from build123d import *

# Parameters (mm, degrees)
SKETCH1_W           = 3
SKETCH1_H           = 3
SKETCH1_H_2         = 54.4
SKETCH1_W_2         = 30.6
SKETCH1_W_3         = 5.5
SKETCH1_W_4         = 13.6
SKETCH1_W_5         = 18
BOSS_EXTRUDE3_DEPTH = 3
SKETCH1_9_W         = 5.5
SKETCH1_9_H         = 3
SKETCH1_9_W_2       = 13.6
SKETCH1_9_W_3       = 18
SKETCH1_9_W_4       = 3
SKETCH1_9_H_2       = 54.4
SKETCH1_9_W_5       = 30.6
BOSS_EXTRUDE4_DEPTH = 15
CUT_EXTRUDE1_DEPTH  = 3
CUT_EXTRUDE2_DEPTH  = 3
SKETCH4_W           = 13.6
SKETCH4_H           = 11
CUT_EXTRUDE3_DEPTH  = 3
CUT_EXTRUDE4_DEPTH  = 3


with BuildPart() as part:
    # Sketch1 → Boss-Extrude3 (new body)
    with BuildSketch(Plane.XY):
        with Locations((1.5, 58.9)):
            Rectangle(SKETCH1_W, SKETCH1_H)
        with Locations((1.5, 30.2)):
            Rectangle(SKETCH1_W, SKETCH1_H_2)
        Polygon((0, 3), (0, 0), (76.2, 0), (76.2, 3), (3, 3), align=None)
        Polygon((3, 3), (76.2, 3), (76.2, 46.2), (58.2, 46.2), (58.2, 29), (52.7, 29), (52.7, 61.4), (39.1, 61.4), (39.1, 29), (33.6, 29), (33.6, 57.4), (3, 57.4), align=None)
        with Locations((18.3, 58.9)):
            Rectangle(SKETCH1_W_2, SKETCH1_H)
        Polygon((33.6, 60.4), (33.6, 57.4), (33.6, 29), (39.1, 29), (39.1, 61.4), (33.6, 61.4), align=None)
        with Locations((36.35, 62.9)):
            Rectangle(SKETCH1_W_3, SKETCH1_H)
        with Locations((45.9, 62.9)):
            Rectangle(SKETCH1_W_4, SKETCH1_H)
        with Locations((55.45, 62.9)):
            Rectangle(SKETCH1_W_3, SKETCH1_H)
        Polygon((58.2, 29), (58.2, 46.2), (58.2, 49.2), (58.2, 61.4), (52.7, 61.4), (52.7, 29), align=None)
        with Locations((67.2, 47.7)):
            Rectangle(SKETCH1_W_5, SKETCH1_H)
        with Locations((77.7, 47.7)):
            Rectangle(SKETCH1_W, SKETCH1_H)
        Polygon((76.2, 3), (76.2, 0), (79.2, 0), (79.2, 46.2), (76.2, 46.2), align=None)
    extrude(amount=BOSS_EXTRUDE3_DEPTH)

    # Sketch1_9 → Boss-Extrude4 (add)
    with BuildSketch(Plane.XY):
        Polygon((33.6, 60.4), (33.6, 57.4), (33.6, 29), (39.1, 29), (39.1, 61.4), (33.6, 61.4), align=None)
        with Locations((36.35, 62.9)):
            Rectangle(SKETCH1_9_W, SKETCH1_9_H)
        with Locations((45.9, 62.9)):
            Rectangle(SKETCH1_9_W_2, SKETCH1_9_H)
        with Locations((55.45, 62.9)):
            Rectangle(SKETCH1_9_W, SKETCH1_9_H)
        Polygon((58.2, 29), (58.2, 46.2), (58.2, 49.2), (58.2, 61.4), (52.7, 61.4), (52.7, 29), align=None)
        with Locations((67.2, 47.7)):
            Rectangle(SKETCH1_9_W_3, SKETCH1_9_H)
        with Locations((77.7, 47.7)):
            Rectangle(SKETCH1_9_W_4, SKETCH1_9_H)
        Polygon((76.2, 3), (76.2, 0), (79.2, 0), (79.2, 46.2), (76.2, 46.2), align=None)
        Polygon((0, 3), (0, 0), (76.2, 0), (76.2, 3), (3, 3), align=None)
        with Locations((1.5, 30.2)):
            Rectangle(SKETCH1_9_W_4, SKETCH1_9_H_2)
        with Locations((18.3, 58.9)):
            Rectangle(SKETCH1_9_W_5, SKETCH1_9_H)
        with Locations((1.5, 58.9)):
            Rectangle(SKETCH1_9_W_4, SKETCH1_9_H)
    extrude(amount=-BOSS_EXTRUDE4_DEPTH)

    # Sketch2 → Cut-Extrude1 (cut)
    with BuildSketch(Plane(origin=(0, 0, 0), x_dir=(-1, 0, 0), z_dir=(0, -1, 0))):
        Polygon((0, 0), (0, 15), (-33.6, 15), (-18.6, 0), align=None)
    extrude(amount=-CUT_EXTRUDE1_DEPTH, mode=Mode.SUBTRACT)

    # Sketch3 → Cut-Extrude2 (cut)
    with BuildSketch(Plane.ZY):
        Polygon((0, 3), (-15, 18), (-15, 3), align=None)
    extrude(amount=-CUT_EXTRUDE2_DEPTH, mode=Mode.SUBTRACT)

    # Sketch4 → Cut-Extrude3 (cut)
    with BuildSketch(Plane(origin=(0, 64.4, 0), x_dir=(1, 0, 0), z_dir=(0, 1, 0))):
        with Locations((45.9, 9.5)):
            Rectangle(SKETCH4_W, SKETCH4_H)
    extrude(amount=-CUT_EXTRUDE3_DEPTH, mode=Mode.SUBTRACT)

    # Sketch5 → Cut-Extrude4 (cut)
    with BuildSketch(Plane(origin=(0, 0, 0), x_dir=(-1, 0, 0), z_dir=(0, -1, 0))):
        Polygon((-33.6, 15), (-51.6, 15), (-36.6, 0), (-18.6, 0), align=None)
    extrude(amount=-CUT_EXTRUDE4_DEPTH, mode=Mode.SUBTRACT)


solid = part.part
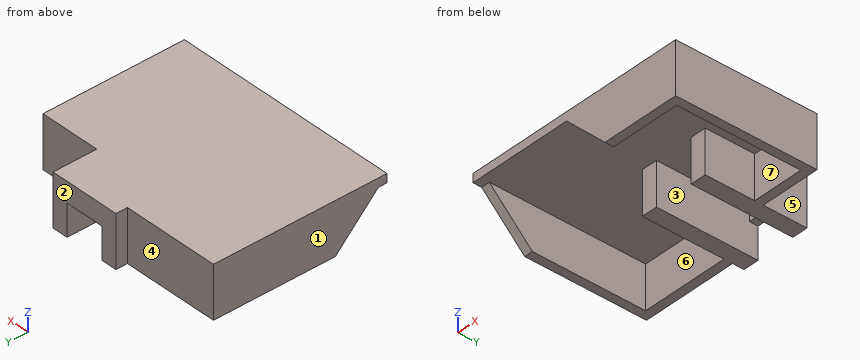
Verification items for the finished model (mm, model axes). Face numbers are marked on the shaded views. A direction names the side the tool comes from. Coordinates: 2 decimals unless noted, no trailing zeros. Order: outer loops, then holes, each group sorted by start corner. A loop starts at its lowest first (then second) coordinate and runs counter-clockwise, first axis right, second up. Notation, with made-up numbers: M 58,-30.5 L 65,-30.5 A15 cw 65,-2.5 Z; hole C 51.25,36.5 d2. An arc over 180 degrees is marked long. Return JSON: item names as keys, results as strings.
1) Thickness scan on L1, parallel to X at y = 30.5, z = -9.25; L2, parallel to X at y = 53.5, z = -0.75; L3, parallel to X at y = 22, z = -3.25. Record the ranges inside material, lowest first. Write a range as [from, to].
Answer list:
{"L1": "[0, 3], [33.6, 39.1], [52.7, 58.2], [76.2, 79.2]", "L2": "[0, 3], [33.6, 39.1], [52.7, 58.2]", "L3": "[0, 3], [76.2, 79.2]"}
2) Release check for a two-part mould opening along X. For the marked faces 1, 2 and 3 record: +X half, -X half, draft (parallel to the pull), parting line (faces both ways), or undercut.
Answer list:
{"face 1": "-X half", "face 2": "draft", "face 3": "undercut"}
3) Access from +Z, -Z, +X, -X, +Y, -Y to the whole of each face (thin tool, end or side, straight path). Record for the marked faces 4, 5, 6 and 7.
Answer list:
{"face 4": "+Z, -Z, -X, +Y", "face 5": "+Z, -Z, +X, +Y", "face 6": "-Z, -Y", "face 7": "-Z"}
4) Cross-section at B-B, the plane y = 22. Record the boundary of the cut face in (x, z).
Answer list:
{"outline": "M 0,-15 L 3,-15 L 3,0 L 76.2,0 L 76.2,-15 L 79.2,-15 L 79.2,3 L 0,3 Z"}
5) Cross-section at D-D, the plane z = -1.75. Record the boundary of the cut face in (x, y).
Answer list:
{"outline": "M 0,4.75 L 3,4.75 L 3,57.4 L 33.6,57.4 L 33.6,29 L 39.1,29 L 39.1,61.4 L 52.7,61.4 L 52.7,29 L 58.2,29 L 58.2,46.2 L 76.2,46.2 L 76.2,3 L 38.35,3 L 38.35,0 L 79.2,0 L 79.2,49.2 L 58.2,49.2 L 58.2,64.4 L 33.6,64.4 L 33.6,60.4 L 0,60.4 Z"}
6) Cross-section at C-C, the plane x = 40.5. Record the boundary of the cut face in (y, z).
Answer list:
{"outline": "M 0,-3.9 L 3,-3.9 L 3,0 L 61.4,0 L 61.4,-4 L 64.4,-4 L 64.4,3 L 0,3 Z"}
7) Cross-section at A-A, the plane z = -6.75. Record the boundary of the cut face in (x, y), and give its area (3 significant figures).
Answer list:
{"outline": "M 0,9.75 L 3,9.75 L 3,57.4 L 33.6,57.4 L 33.6,29 L 39.1,29 L 39.1,64.4 L 33.6,64.4 L 33.6,60.4 L 0,60.4 Z; M 43.35,0 L 79.2,0 L 79.2,49.2 L 58.2,49.2 L 58.2,64.4 L 52.7,64.4 L 52.7,29 L 58.2,29 L 58.2,46.2 L 76.2,46.2 L 76.2,3 L 43.35,3 Z", "area": "933 mm2"}
8) Gauge pin test, flat ends, axial feed: pin 1 (3.5 mm diameter, centred on x = 46.5, y = 63.5, fed in from -Z); pin 2 (1.5 mm diameter, centred on x = 11.5, z = -10, fed in from -Y); pin 3 (6 mm diameter, centred on x = 36, z = -9, fed in from -Y). Record the tip position at first contact, or that the pin passes through.
Answer list:
{"pin 1": "z = -4", "pin 2": "y = 57.4", "pin 3": "y = 29"}
